```python
from build123d import *

# Parameters (mm, degrees)
SKETCH4_R                                            = 5.5
SKETCH4_R_2                                          = 3
BOSS_EXTRUDE2_DEPTH                                  = 10
CSK_FOR_M6_HEX_SOCKET_COUNTERSUNK_CAP_SC_D           = 6.3
CSK_FOR_M6_HEX_SOCKET_COUNTERSUNK_CAP_SC_CSINK_D     = 12.5
CSK_FOR_M6_HEX_SOCKET_COUNTERSUNK_CAP_SC_CSINK_ANGLE = 90
SKETCH7_R                                            = 6.65
CUT_EXTRUDE1_DEPTH                                   = 5.3
SKETCH8_R                                            = 12.75
CUT_EXTRUDE2_DEPTH                                   = 3


with BuildPart() as part:
    # Sketch4 → Boss-Extrude2 (new body)
    with BuildSketch(Plane.XY):
        with BuildLine():
            Line((9.292402207, 1.975161063), (-1.224202506, 51.451896246))
            ThreePointArc((-1.224202506, 51.451896246), (-39.996949985, 32.388891475), (-50.582074879, -9.5))
            Line((-50.582074879, -9.5), (0, -9.5))
            ThreePointArc((0, -9.5), (7.382886634, -5.978543715), (9.292402207, 1.975161063))
        make_face()
        Circle(SKETCH4_R, mode=Mode.SUBTRACT)
        with Locations((-27.951187583, 22.634425413)):
            Circle(SKETCH4_R_2, mode=Mode.SUBTRACT)
    extrude(amount=BOSS_EXTRUDE2_DEPTH)

    # CSK for M6 Hex Socket Countersunk Cap Screw1 (through all)
    with Locations(Plane(origin=(0, 0, 0), x_dir=(-1, 0, 0), z_dir=(0, 0, -1))):
        with Locations((27.951187583, 22.634425413)):
            CounterSinkHole(CSK_FOR_M6_HEX_SOCKET_COUNTERSUNK_CAP_SC_D / 2, CSK_FOR_M6_HEX_SOCKET_COUNTERSUNK_CAP_SC_CSINK_D / 2, counter_sink_angle=CSK_FOR_M6_HEX_SOCKET_COUNTERSUNK_CAP_SC_CSINK_ANGLE)

    # Sketch7 → Cut-Extrude1 (cut)
    with BuildSketch(Plane(origin=(0, 0, 0), x_dir=(-1, 0, 0), z_dir=(0, 0, -1))):
        Circle(SKETCH7_R)
    extrude(amount=-CUT_EXTRUDE1_DEPTH, mode=Mode.SUBTRACT)

    # Sketch8 → Cut-Extrude2 (cut)
    with BuildSketch(Plane.XY.offset(10)):
        with Locations((-27.951187583, 22.634425413)):
            Circle(SKETCH8_R)
    extrude(amount=-CUT_EXTRUDE2_DEPTH, mode=Mode.SUBTRACT)


solid = part.part
```
Work out the finished part from the listing and answer in its coordinate system (mm). A direction names the side the tool comes from. Give positions to 0.01 mm unless a question says otherwise; leave off trailing zeros. Loops run counter-clockwise (first coordinate to the right, second up) from the corner with the lowest first, then second, coordinate; pieces in that order, holes last. Notation, with made-up numbers: (88.25, 29) - (104.25, 29) arc R8 ccw to (104.25, 35) - close; hole circle Ø5 at (81, 88.5). An arc over 180 degrees is marked (long way). Use CSV: the item, a comma, the result in double quotes. Start each with the question number.
(1) Determine the mould class of faces 4 (the face through (4.1, 26.4, 4.9)), 5 (the face through (-25, 20, 7)), 6 (the face through (-21, 15, 0)) for opening direction X: released by +X, released by -X, zero draft, split by the parting line, or undercut.
(2) Find section D-D, the plane x = -44. Determine the outline of the cut face in (y, z), plus the area to 3 significant figures.
(3) A tool of negligible diameter and unlimited length cuts with its end or side. For faces 1 (the face through (-22.07, 11.32, 8.52)), 2 (the face through (-3.07, -5.9, 2.61)), 3 (the face through (-26, -9.5, 5)), from which of +Z, -Z, +X, -X, +Y, -Y can it reach the whole face along a straight path? Write none if from no direction.
(4) Find section B-B, the plane z = 8. Determine the outline of the cut face in (x, y), plus the area to 3 significant figures.
(5) Find section C-C, the plane y = 30.5. Determine the outline of the cut face in (x, z).
(6) Find the intervals of material crossed by L1, parallel to X at y = 0, z = 6.35; L2, parallel to X at y = 23, z = 4.5; L3, parallel to Y at x = -34.5, z = 7.5, in increasing order.
(7) Find section A-A, the plane y = 0. Determine the outline of the cut face in (x, z).
(8) Each of these flat-tipped pins is pushed along its axis until it touches: pin 1 (10 mm diameter, centred on x = -27.95, y = 22.63, fed in from -Z); pin 2 (4 mm diameter, centred on x = 3, y = -1, fed in from -Z); pin 3 (12 mm diameter, centred on x = 0, y = 0, fed in from -Z); pin 4 (6 mm diameter, centred on y = 9.5, z = 9, fed in from +X). Where does it stop, or does it pass through?
Results found:
1,face 4,"released by +X"
1,face 5,"undercut"
1,face 6,"zero draft"
2,outline,"(-9.5, 0) - (26.7, 0) - (26.7, 10) - (-9.5, 10) - close"
2,area,"362 mm^2"
3,face 1,"+Z"
3,face 2,"-Z"
3,face 3,"+Z, -Z, +X, -X, -Y"
4,outline,"(-50.58, -9.5) - (0, -9.5) arc R9.5 ccw to (9.29, 1.98) - (-1.22, 51.45) arc R51.47 ccw to start; hole circle Ø25.5 at (-27.95, 22.63); hole circle Ø11 at (0, 0)"
4,area,"2,250 mm^2"
5,outline,"(-41.46, 0) - (3.23, 0) - (3.23, 10) - (-17.92, 10) - (-17.92, 7) - (-37.99, 7) - (-37.99, 10) - (-41.46, 10) - close"
6,L1,"-51.47 to -5.5, 5.5 to 9.5"
6,L2,"-46.04 to -31.08, -24.82 to 4.82"
6,L3,"-9.5 to 11.69, 33.57 to 38.19"
7,outline,"(-51.47, 0) - (-6.65, 0) - (-6.65, 5.3) - (-5.5, 5.3) - (-5.5, 10) - (-51.47, 10) - close; (5.5, 5.3) - (6.65, 5.3) - (6.65, 0) - (9.5, 0) - (9.5, 10) - (5.5, 10) - close"
8,pin 1,"z = 1.25"
8,pin 2,"through"
8,pin 3,"z = 5.3"
8,pin 4,"x = 8.33"
